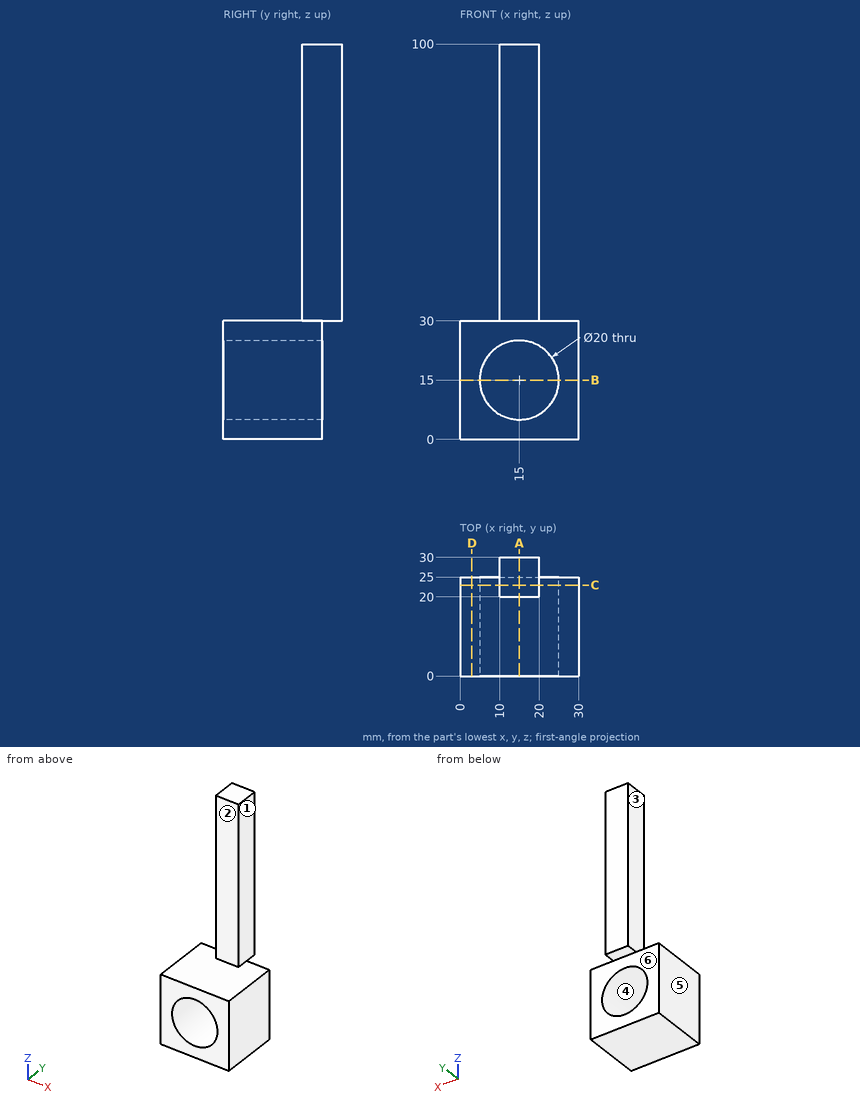
Geometry check sheet. Reference: drawing and pictorial views, mm from the part's lowest x, y, z. A direction names the side the tool comes from. Round coordinates to 2 decimals unless told otherwise and drop trailing zeros. Loops run counter-clockwise (first coordinate to the right, second up) from the corner with the lowest first, then second, coordinate; pieces in that order, holes last.
1. Scan lines: probe 1 along Z at (x, y) = (15, 17.25); probe 2 along Z at (x, y) = (12.25, 15.5); probe 3 along Y at (x, z) = (19, 95). Record each from-to range of solid material in increasing order.
2. Sectioned sample at A-A on x = 15. Record the boundary of the cut face in (y, z).
3. Sectioned sample at C-C on y = 23. Record the boundary of the cut face in (x, z).
4. Mould release check, pull along X, two halves, no side actions. Record for the marked faces 4, 5 and 6: released by +X, released by -X, zero draft, split by the parting line, or undercut.
5. Set-up check for the marked faces 1, 2 and 3: record each of +Z, -Z, +X, -X, +Y, -Y from which the full face is reachable in a straight line by a thin tool's end or side.
6. Gauge pin test, flat ends, axial feed: pin 1 Ø5 at (x, y) = (18.5, 8.5) entering from -Z; pin 2 Ø12.5 at (x, y) = (16, 7.5) entering from +Z; pin 3 Ø8 at (y, z) = (27, 65.5) entering from -X; pin 4 Ø8 at (y, z) = (22.5, 64.5) entering from +X. Record the tip position at first contact, or that the pin passes through.
7. Sectioned sample at B-B on z = 15. Record the boundary of the cut face in (x, y), and give its area (3 significant figures).
8. Sectioned sample at D-D on x = 3. Record the boundary of the cut face in (y, z), and give its area (3 significant figures).
Recorded:
1. probe 1: z = 0 to 5, 25 to 30
1. probe 2: z = 0 to 5.39, 24.61 to 30
1. probe 3: y = 20 to 30
2. outline: (0, 0) - (25, 0) - (25, 5) - (0, 5) - close; (0, 25) - (25, 25) - (25, 30) - (30, 30) - (30, 100) - (20, 100) - (20, 30) - (0, 30) - close
3. outline: (0, 0) - (30, 0) - (30, 30) - (20, 30) - (20, 100) - (10, 100) - (10, 30) - (0, 30) - close; hole circle Ø20 at (15, 15)
4. face 4: undercut
4. face 5: released by -X
4. face 6: zero draft
5. face 1: +Z, +X, +Y, -Y
5. face 2: +Z, +X, -X, -Y
5. face 3: +Z, -X, +Y, -Y
6. pin 1: stops at z = 0
6. pin 2: stops at z = 30
6. pin 3: stops at x = 10
6. pin 4: stops at x = 20
7. outline: (0, 0) - (5, 0) - (5, 25) - (0, 25) - close; (25, 0) - (30, 0) - (30, 25) - (25, 25) - close
7. area: 250 mm2
8. outline: (0, 0) - (25, 0) - (25, 30) - (0, 30) - close
8. area: 750 mm2
